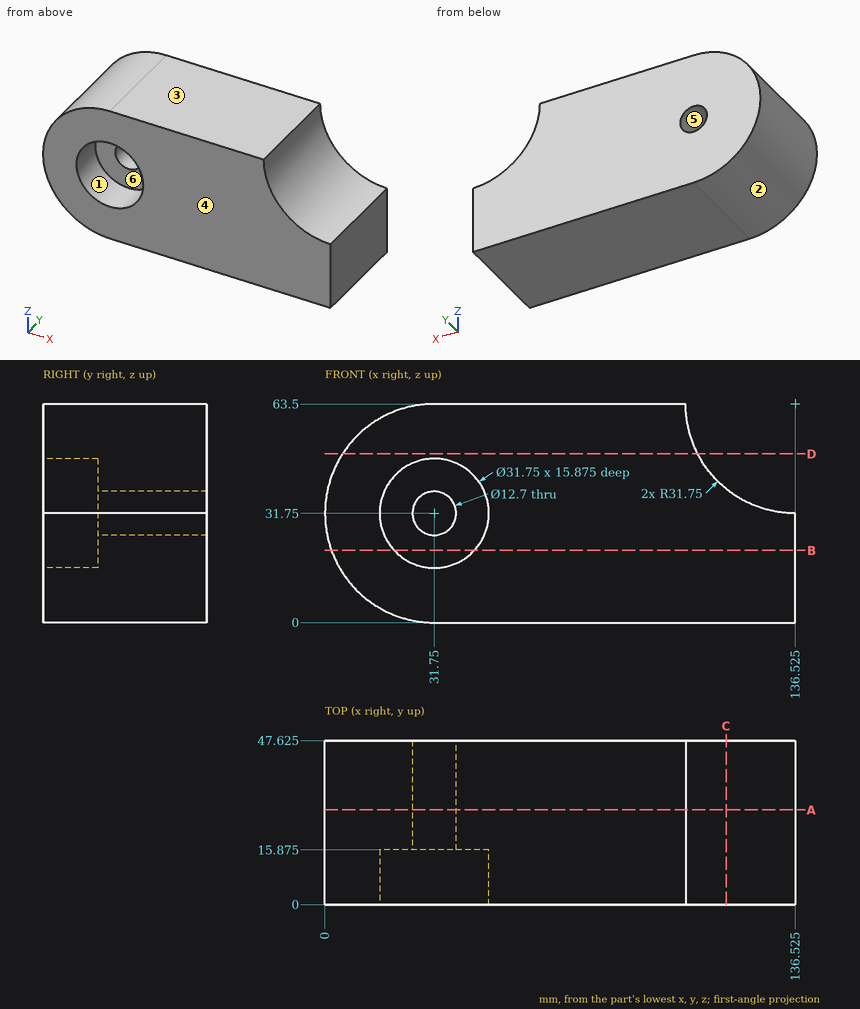
Study the drawing (mm; zero at the part's minimum x, y, z) and answer. A direction names the side the tool comes from. Coordinates: 2 decimals unless noted, no trailing zeros. Loops run counter-clockwise (first coordinate to the right, second up) from the corner with the lowest first, then second, coordinate; pieces in that order, holes last. Notation, with made-up numbers: M 3,36 L 14,36 A24 ccw 14,47 Z; hole C -14.5,27 d5. An arc over 180 degrees is marked long. Answer in a Markdown table with one row per item.
1) Find section A-A (y = 27.5). Determine the outline of the cut face in (x, z) (3 decimals), then the cut area to 3 significant figures.
Answers below:
| item | result |
|---|---|
| outline | M 31.75,0 L 136.525,0 L 136.525,31.75 A31.75 cw 104.775,63.5 L 31.75,63.5 A31.75 ccw Z; hole C 31.75,31.75 d12.7 |
| area | 7,320 mm^2 |
2) Which of the six approach directions +Z, -Z, +X, -X, +Y, -Y give full straight-line access (tool end or side, diameter ignored) to the marked faces 1 and 2?
Answers below:
| item | result |
|---|---|
| face 1 | -Y |
| face 2 | -X, +Y, -Y |
3) Find section D-D (z = 49). Determine the outline of the cut face in (x, y) (3 decimals).
Answers below:
| item | result |
|---|---|
| outline | M 5.095,0 L 108.279,0 L 108.279,47.625 L 5.095,47.625 Z |
4) Determine the mould class of the marked faces 3, 4, 5 and 6 for opening direction Z: released by +Z, released by -Z, zero draft, split by the parting line, or undercut.
Answers below:
| item | result |
|---|---|
| face 3 | released by +Z |
| face 4 | zero draft |
| face 5 | undercut |
| face 6 | undercut |
5) Find section B-B (z = 21). Determine the outline of the cut face in (x, y) (3 decimals).
Answers below:
| item | result |
|---|---|
| outline | M 1.875,0 L 20.069,0 L 20.069,15.875 L 43.431,15.875 L 43.431,0 L 136.525,0 L 136.525,47.625 L 1.875,47.625 Z |
6) Find section C-C (x = 116.5). Determine the outline of the cut face in (y, z) (3 decimals), then the cut area to 3 significant figures.
Answers below:
| item | result |
|---|---|
| outline | M 0,0 L 47.625,0 L 47.625,38.861 L 0,38.861 Z |
| area | 1,850 mm^2 |
7) Find the intervals of material crossed by probe 1 along Z at (x, y) = (31.75, 4) (3 decimals); probe 2 along Z at (x, y) = (31, 23); probe 3 along X at (y, z) = (28, 36), in increasing order.
Answers below:
| item | result |
|---|---|
| probe 1 | 0 to 15.875, 47.625 to 63.5 |
| probe 2 | 0.01 to 25.44, 38.06 to 63.49 |
| probe 3 | 0.29 to 27.03, 36.47 to 120.66 |
8) Given pin 1 (1.5 mm diameter, centred on x = 60, z = 39.5, fed in from -Y); pin 2 (6 mm diameter, centred on x = 18, y = 7, fed in from -Z); pin 3 (5 mm diameter, centred on y = 24, z = 35, fed in from -X), each flat-ended and moving along its own axis, determine where each tip first touches the part or whether it passes through.
Answers below:
| item | result |
|---|---|
| pin 1 | y = 0 |
| pin 2 | z = 1.88 |
| pin 3 | x = 0.01 |
